CAD build for the part. Positions are in the model's coordinates, mm. Face numbers are marked on the shaded views. A direction names the side the tool comes from. Round coordinates to 2 decimals unless told otherwise and drop trailing zeros. Loops run counter-clockwise (first coordinate to the right, second up) from the corner with the lowest first, then second, coordinate; pieces in that order, holes last.
```python
from build123d import *

# Parameters (mm, degrees)
SKETCH1_W               = 11.9888
SKETCH1_H               = 14.986
BOSS_EXTRUDE1_DEPTH     = 3.175
SKETCH6_W               = 25.1714
SKETCH6_H               = 14.986
BOSS_EXTRUDE6_DEPTH     = 3.175
SKETCH10_W              = 24.6888
SKETCH10_H              = 14.986
BOSS_EXTRUDE7_DEPTH     = 3.175
M3_CLEARANCE_HOLE1_D    = 3.2
SKETCH15_R              = 0.79375
CUT_EXTRUDE5_DEPTH      = 41.467708539
CUT_EXTRUDE6_DEPTH      = 1.5875
SKETCH17_W              = 9.525
SKETCH17_H              = 14.986
BOSS_EXTRUDE8_DEPTH     = 12.7
CUT_EXTRUDE7_DEPTH      = 2.38125
CUT_EXTRUDE7_DEPTH_BACK = 2.38125
SKETCH19_W              = 12.7
SKETCH19_H              = 14.986
SKETCH20_R              = 1.5875
CUT_EXTRUDE8_DEPTH      = 16.60525
CUT_EXTRUDE9_DEPTH      = 3.39725


with BuildPart() as part:
    # Sketch1 → Boss-Extrude1 (new body)
    with BuildSketch(Plane.XY):
        with Locations((5.9944, 7.493)):
            Rectangle(SKETCH1_W, SKETCH1_H)
    extrude(amount=BOSS_EXTRUDE1_DEPTH)

    # Sketch6 → Boss-Extrude6 (add)
    with BuildSketch(Plane(origin=(11.9888, 0, 0), x_dir=(0, 0, -1), z_dir=(1, 0, 0))):
        with Locations((-12.5857, 7.493)):
            Rectangle(SKETCH6_W, SKETCH6_H)
    extrude(amount=BOSS_EXTRUDE6_DEPTH)

    # Sketch10 → Boss-Extrude7 (add)
    with BuildSketch(Plane.XY.offset(25.1714)):
        with Locations((12.3444, 7.493)):
            Rectangle(SKETCH10_W, SKETCH10_H)
    extrude(amount=BOSS_EXTRUDE7_DEPTH)

    # M3 Clearance Hole1 (through all)
    with Locations(Plane(origin=(-0.089803774, -1.114373232, 0), x_dir=(1, 0, 0), z_dir=(0, 0, -1))):
        with Locations((6.084203774, -12.112573232), (6.084203774, -5.102173232)):
            Hole(M3_CLEARANCE_HOLE1_D / 2)

    # Sketch15 → Cut-Extrude5 (cut, through all)
    with BuildSketch(Plane.XZ):
        with Locations((11.9888, 25.1714)):
            Circle(SKETCH15_R)
        with Locations((11.9888, 3.175)):
            Circle(SKETCH15_R)
    extrude(amount=-CUT_EXTRUDE5_DEPTH, mode=Mode.SUBTRACT)

    # Sketch16 → Cut-Extrude6 (cut)
    with BuildSketch(Plane(origin=(0, 0, 0), x_dir=(-1, 0, 0), z_dir=(0, 0, -1))):
        Polygon((-4.40668676, 6.7378), (-7.58211324, 6.7378), (-9.169826481, 3.9878), (-7.58211324, 1.2378), (-4.40668676, 1.2378), (-2.818973519, 3.9878), align=None)
        Polygon((-4.40668676, 13.7482), (-7.58211324, 13.7482), (-9.169826481, 10.9982), (-7.58211324, 8.2482), (-4.40668676, 8.2482), (-2.818973519, 10.9982), align=None)
    extrude(amount=-CUT_EXTRUDE6_DEPTH, mode=Mode.SUBTRACT)

    # Sketch17 → Boss-Extrude8 (add)
    with BuildSketch(Plane(origin=(0, 0, 25.1714), x_dir=(-1, 0, 0), z_dir=(0, 0, -1))):
        with Locations((-19.9263, 7.493)):
            Rectangle(SKETCH17_W, SKETCH17_H)
    extrude(amount=BOSS_EXTRUDE8_DEPTH)

    # Sketch19 → Cut-Extrude7 (cut, two sides: drawn at the far end of the back side and taken through both)
    with BuildSketch(Plane(origin=(19.9263, 0, 0), x_dir=(0, 0, -1), z_dir=(1, 0, 0)).offset(-CUT_EXTRUDE7_DEPTH_BACK)):
        with Locations((-18.8214, 7.493)):
            Rectangle(SKETCH19_W, SKETCH19_H)
    extrude(amount=CUT_EXTRUDE7_DEPTH + CUT_EXTRUDE7_DEPTH_BACK, mode=Mode.SUBTRACT)

    # Sketch20 → Cut-Extrude8 (cut)
    with BuildSketch(Plane(origin=(24.6888, 0, 0), x_dir=(0, 0, -1), z_dir=(1, 0, 0))):
        with Locations((-18.8214, 7.493)):
            Circle(SKETCH20_R)
    extrude(amount=-CUT_EXTRUDE8_DEPTH, mode=Mode.SUBTRACT)

    # Sketch21 → Cut-Extrude9 (cut)
    with BuildSketch(Plane.ZY.offset(-11.9888)):
        Polygon((22.487574209, 7.493), (20.654487105, 10.668), (16.988312895, 10.668), (15.155225791, 7.493), (16.988312895, 4.318), (20.654487105, 4.318), align=None)
    extrude(amount=-CUT_EXTRUDE9_DEPTH, mode=Mode.SUBTRACT)


solid = part.part
```
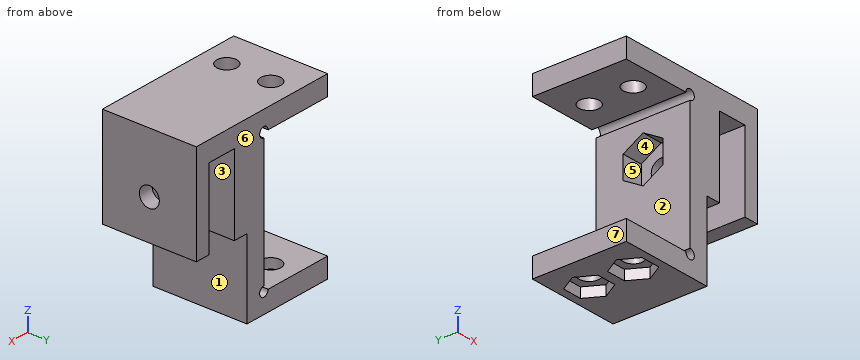
Item 1: Flat gauge pins, fed straight in: P1, Ø5, axis at x = 19.5, y = 6.5, coming from the -Z side; P2, Ø1.5, axis at x = 6, z = 3.5, coming from the -Y side; P3, Ø1.5, axis at y = 4.5, z = 14.5, coming from the -X side; P4, Ø2, axis at y = 5.5, z = 10, coming from the +X side. Where does each tip first touch, or does it go through?
Answers follow:
P1: stops at z = 12.47
P2: stops at y = 0
P3: stops at x = 11.99
P4: stops at x = 15.16
Item 2: Cut at D-D, the plane y = 4.75. State how many separate pieces and enclosed holes the cut face has, plus the area to 3 significant figures.
Answers follow:
separate pieces: 3
enclosed holes: 0
area: 218 mm2
Item 3: Cut at C-C, the plane z = 18.5. Give the cut face in (x, y).
Answers follow:
outline: (11.99, 0) - (17.55, 0) - (17.55, 5.94) - (15.39, 5.94) - (15.39, 4.32) - (11.99, 4.32) - close; (11.99, 10.67) - (15.39, 10.67) - (15.39, 9.05) - (17.55, 9.05) - (17.55, 14.99) - (11.99, 14.99) - close; (22.31, 0) - (24.69, 0) - (24.69, 5.94) - (22.31, 5.94) - close; (22.31, 9.05) - (24.69, 9.05) - (24.69, 14.99) - (22.31, 14.99) - close
Item 4: Two-plate mould, pull along Y, no slides. Class the marked faces 5, 6 and 7: released by +Y, released by -Y, zero draft, split by the parting line, or undercut.
Answers follow:
face 5: undercut
face 6: released by +Y
face 7: zero draft
Item 5: 3-axis set-ups, long thin cutter, end or side, ignore diameter. For the marked faces 1, 2, 3 and 4: which of +Z, -Z, +X, -X, +Y, -Y reach the whole face in a straight line?
Answers follow:
face 1: -Z, +X, +Y, -Y
face 2: -X, +Y, -Y
face 3: -Z, +Y, -Y
face 4: -X
Item 6: Cut at B-B, the plane x = 13.5. Give the cut face in (y, z), plus the area to 3 significant figures.
Answers follow:
outline: (0, 0) - (14.99, 0) - (14.99, 28.35) - (0, 28.35) - close; hole (4.32, 16.99) - (7.49, 15.16) - (10.67, 16.99) - (10.67, 20.65) - (7.49, 22.49) - (4.32, 20.65) - close
area: 390 mm2
Item 7: Probe line 1 (X direction, y = 12.25, z = 17); line 2 (X direction, y = 9.75, z = 21); line 3 (X direction, y = 4.5, z = 2.75). List the from-to ranges inside material, lowest first.
Answers follow:
line 1: x = 11.99 to 17.55, 22.31 to 24.69
line 2: x = 15.39 to 17.55, 22.31 to 24.69
line 3: x = 0 to 4.48, 7.51 to 11.32, 12.66 to 15.16
Item 8: Cut at A-A, the plane x = 2. Give the cut face in (y, z) (3 decimals), plus the area to 3 significant figures.
Answers follow:
outline: (0, 0) - (14.986, 0) - (14.986, 3.175) - (0, 3.175) - close; (0, 25.171) - (14.986, 25.171) - (14.986, 28.346) - (0, 28.346) - close
area: 95.2 mm2
